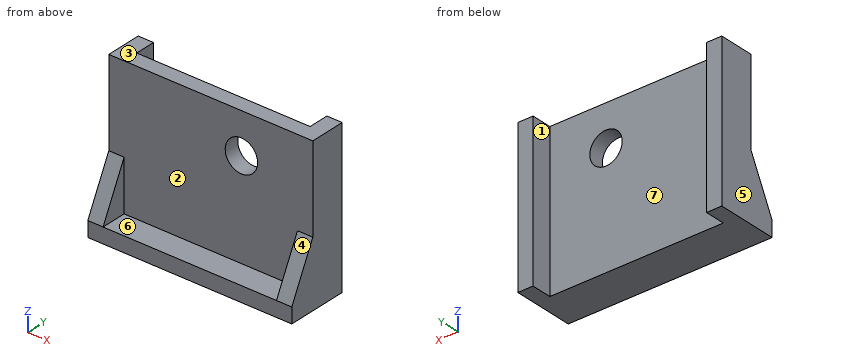
```python
from build123d import *

# Parameters (mm, degrees)
SKETCH1_W           = 40
SKETCH1_H           = 30
BOSS_EXTRUDE2_DEPTH = 3
SKETCH2_W           = 3
SKETCH2_H           = 30
BOSS_EXTRUDE3_DEPTH = 4
SKETCH3_W           = 3
SKETCH3_H           = 30
BOSS_EXTRUDE4_DEPTH = 4
SKETCH4_R           = 3.175
CUT_EXTRUDE1_DEPTH  = 43.489507814
SKETCH5_W           = 40
SKETCH5_H           = 3
BOSS_EXTRUDE5_DEPTH = 5
RIB4_REACH          = 50.765
SKETCH8_WALL_W      = 110.70982261
SKETCH8_WALL_H      = 3
RIB5_REACH          = 50.765
SKETCH10_WALL_W     = 110.70982261
SKETCH10_WALL_H     = 3


with BuildPart() as part:
    # Sketch1 → Boss-Extrude2 (new body)
    with BuildSketch(Plane(origin=(0, 0, 0), x_dir=(1, 0, 0), z_dir=(0, 1, 0))):
        with Locations((-19.478413565, 0.192535557)):
            Rectangle(SKETCH1_W, SKETCH1_H)
    extrude(amount=BOSS_EXTRUDE2_DEPTH)

    # Sketch2 → Boss-Extrude3 (add)
    with BuildSketch(Plane(origin=(0, 3, 0), x_dir=(1, 0, 0), z_dir=(0, 1, 0))):
        with Locations((-0.978413565, 0.192535557)):
            Rectangle(SKETCH2_W, SKETCH2_H)
    extrude(amount=BOSS_EXTRUDE3_DEPTH)

    # Sketch3 → Boss-Extrude4 (add)
    with BuildSketch(Plane(origin=(0, 3, 0), x_dir=(1, 0, 0), z_dir=(0, 1, 0))):
        with Locations((-37.978413565, 0.192535557)):
            Rectangle(SKETCH3_W, SKETCH3_H)
    extrude(amount=BOSS_EXTRUDE4_DEPTH)

    # Sketch4 → Cut-Extrude1 (cut, through all)
    with BuildSketch(Plane(origin=(0, 3, 0), x_dir=(1, 0, 0), z_dir=(0, 1, 0))):
        with Locations(Location((-13.478413565, -6.807464443, 0), (0, 0, 270))):
            Circle(SKETCH4_R)
    extrude(amount=-CUT_EXTRUDE1_DEPTH, mode=Mode.SUBTRACT)

    # Sketch5 → Boss-Extrude5 (add)
    with BuildSketch(Plane(origin=(0, 0, 0), x_dir=(-1, 0, 0), z_dir=(0, -1, 0))):
        with Locations((19.478413565, 13.692535557)):
            Rectangle(SKETCH5_W, SKETCH5_H)
    extrude(amount=BOSS_EXTRUDE5_DEPTH)

    # Sketch8 wall → Rib4 (add, up to next)
    with BuildSketch(Plane(origin=(0.521586435, -2.5, -7.192535557), x_dir=(0, 0.4472135955, 0.894427191), z_dir=(0, 0.894427191, -0.4472135955)), mode=Mode.PRIVATE) as rib4_sk1:
        with Locations((0, -1.5)):
            Rectangle(SKETCH8_WALL_W, SKETCH8_WALL_H)
    rib4_tool1 = extrude(rib4_sk1.sketch, amount=RIB4_REACH, mode=Mode.PRIVATE) - part.part
    add(rib4_tool1.solids().sort_by_distance((0.521586435, -2.5, -7.192535557))[0])

    # Sketch10 wall → Rib5 (add, up to next)
    with BuildSketch(Plane(origin=(-39.478413565, -2.5, -7.192535557), x_dir=(0, 0.4472135955, 0.894427191), z_dir=(0, 0.894427191, -0.4472135955)), mode=Mode.PRIVATE) as rib5_sk1:
        with Locations((0, 1.5)):
            Rectangle(SKETCH10_WALL_W, SKETCH10_WALL_H)
    rib5_tool1 = extrude(rib5_sk1.sketch, amount=RIB5_REACH, mode=Mode.PRIVATE) - part.part
    add(rib5_tool1.solids().sort_by_distance((-39.478413565, -2.5, -7.192535557))[0])


solid = part.part
```
CAD build for the part. Positions are in the model's coordinates, mm. Face numbers are marked on the shaded views. A direction names the side the tool comes from. Coordinates: 2 decimals unless noted, no trailing zeros. Write each loop counter-clockwise with the first axis right and the second up, starting at its lowest first coordinate (ties: lowest second). Pieces come first, ordered by that corner, then holes.
(1) Cut at D-D, the plane z = 8.75. List the corners of the cut face in (x, y), and give its area (3 significant figures).
(2) Cut at C-C, the plane x = -14.5. List the corners of the cut face in (y, z), and give its area (3 significant figures).
(3) Drill centre lines: probe 1 along X at (y, z) = (6.75, 5.5); probe 2 along Y at (x, z) = (-19, -3); probe 3 along Z at (x, y) = (-25, -0.5). Where is each one in solid material? Low to high.
(4) Two-plate mould, pull along X, no slides. Class the marked faces 4, 5, 6 and 7: +X half, -X half, draft (parallel to the pull), parting line (faces both ways), or undercut.
(5) 3-axis set-ups, long thin cutter, end or side, ignore diameter. For the marked faces 1, 2 and 3: which of +Z, -Z, +X, -X, +Y, -Y reach the whole face in a straight line?
(6) Cut at A-A, the plane y = 4.5. List the corners of the cut face in (x, z).
(7) Cut at B-B, the plane z = 11.75. List the corners of the cut face in (x, y), and give its area (3 significant figures).
(8) Flat gauge pins, fed straight in: pin 1 (2 mm diameter, centred on x = -13, z = 2.5, fed in from -Y); pin 2 (1.5 mm diameter, centred on x = -3.5, z = -7, fed in from +Y); pin 3 (5.5 mm diameter, centred on x = -18, y = -3.5, fed in from +Z). Where does each tip first touch, or does it go through?
Geometry says:
1. outline: (-39.48, 0) - (-15.99, 0) - (-15.99, 3) - (-36.48, 3) - (-36.48, 7) - (-39.48, 7) - close; (-10.97, 0) - (0.52, 0) - (0.52, 7) - (-2.48, 7) - (-2.48, 3) - (-10.97, 3) - close
1. area: 129 mm2
2. outline: (-5, -15.19) - (3, -15.19) - (3, 3.8) - (0, 3.8) - (0, -12.19) - (-5, -12.19) - close; (0, 9.81) - (3, 9.81) - (3, 14.81) - (0, 14.81) - close
2. area: 87.0 mm2
3. probe 1: x = -39.48 to -36.48, -2.48 to 0.52
3. probe 2: y = 0 to 3
3. probe 3: z = -15.19 to -12.19
4. face 4: draft
4. face 5: -X half
4. face 6: undercut
4. face 7: undercut
5. face 1: +Z, -Z, +Y
5. face 2: +Z, -Y
5. face 3: +Z, +X, -X, +Y, -Y
6. outline: (-39.48, -15.19) - (-36.48, -15.19) - (-36.48, 14.81) - (-39.48, 14.81) - close; (-2.48, -15.19) - (0.52, -15.19) - (0.52, 14.81) - (-2.48, 14.81) - close
7. outline: (-39.48, 0) - (0.52, 0) - (0.52, 7) - (-2.48, 7) - (-2.48, 3) - (-36.48, 3) - (-36.48, 7) - (-39.48, 7) - close
7. area: 144 mm2
8. pin 1: stops at y = 0
8. pin 2: stops at y = 3
8. pin 3: stops at z = -12.19
